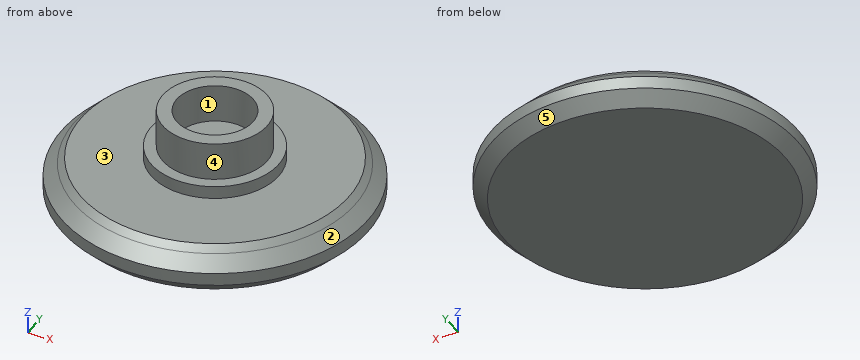
```python
from build123d import *

# Parameters (mm, degrees)
F0_R     = 12
F0_R_2   = 11
F0_R_3   = 5
F0_R_4   = 4.1
F0_R_5   = 3
F1_DEPTH = 2
F2_DEPTH = 3.5
F3_SIZE  = 0.99999
F4_DEPTH = 4.5
F5_DEPTH = 7.5
F6_SIZE  = 1
F7_SIZE  = 0.5


# Not quite as in the source:
# - a fillet or chamfer is up to 0.001 mm smaller than in the source, because OpenCascade refuses the exact size


with BuildPart() as f1:
    # F0 (on Top) → F1 (new body)
    with BuildSketch(Plane.XY):
        Circle(F0_R)
        Circle(F0_R_2, mode=Mode.SUBTRACT)
        Circle(F0_R_2)
        Circle(F0_R_3, mode=Mode.SUBTRACT)
        Circle(F0_R_3)
        Circle(F0_R_4, mode=Mode.SUBTRACT)
        Circle(F0_R_4)
        Circle(F0_R_5, mode=Mode.SUBTRACT)
        Circle(F0_R_5)
    extrude(amount=F1_DEPTH)

    # F0 (on Top) → F2 (join)
    with BuildSketch(Plane.XY):
        Circle(F0_R_2)
        Circle(F0_R_3, mode=Mode.SUBTRACT)
        Circle(F0_R_3)
        Circle(F0_R_4, mode=Mode.SUBTRACT)
        Circle(F0_R_4)
        Circle(F0_R_5, mode=Mode.SUBTRACT)
        Circle(F0_R_5)
    extrude(amount=F2_DEPTH)

    # F3 (size 1 in the source; OpenCascade refuses exactly that, so slightly less here)
    f3_edges = [f1.edges().sort_by_distance(p)[0] for p in [
        (-11, 0, 2),
    ]]
    chamfer(f3_edges, length=F3_SIZE)

    # F0 (on Top) → F4 (join)
    with BuildSketch(Plane.XY):
        Circle(F0_R_3)
        Circle(F0_R_4, mode=Mode.SUBTRACT)
        Circle(F0_R_4)
        Circle(F0_R_5, mode=Mode.SUBTRACT)
        Circle(F0_R_5)
    extrude(amount=F4_DEPTH)

    # F0 (on Top) → F5 (join)
    with BuildSketch(Plane.XY):
        Circle(F0_R_4)
        Circle(F0_R_5, mode=Mode.SUBTRACT)
    extrude(amount=F5_DEPTH)

    # F6
    f6_edges = [f1.edges().sort_by_distance(p)[0] for p in [
        (-12, 0, 0),
    ]]
    chamfer(f6_edges, length=F6_SIZE)

    # F7
    f7_edges = [f1.edges().sort_by_distance(p)[0] for p in [
        (-11, 0, 3.5),
    ]]
    chamfer(f7_edges, length=F7_SIZE)


solid = f1.part
```
Geometry: final body of the model. Coordinates: model frame, mm. Face numbers are marked on the shaded views. A direction names the side the tool comes from. Round coordinates to 2 decimals unless told otherwise and drop trailing zeros. Order: outer loops, then holes, each group sorted by start corner. A loop starts at its lowest first (then second) coordinate and runs counter-clockwise, first axis right, second up. Notation, with made-up numbers: (21, 56.25) - (70, 56.25) arc R30 cw to (70, 85.25) - close; hole circle Ø6 at (33, -37). An arc over 180 degrees is marked (long way). Use CSV: the item, a comma, the result in double quotes. Start each with the question number.
Q1. Access query for the marked faces 4 and 5. Directions: +Z, -Z, +X, -X, +Y, -Y. A direction counts if a zero-diameter tool reaches every point of the face in a straight line with its end or side. Return the directions, or none.
Q2. Material intervals for line 1 along X through (y, z) = (0, 6.4); line 2 along Z through (x, y) = (4.75, -4.5), sorted ascending. Write a range as from..to.
Q3. Section query D-D (z = 4). Return loops of the section in (x, y).
Q4. Mould query, pull axis Y, two halves, no side actions, for the marked faces 1, 2 and 3. Classes: +Y half, -Y half, draft (parallel to the pull), parting line (faces both ways), or undercut.
Q5. Section query B-B (z = 6.75). Return loops of the section in (x, y), and give its area (3 significant figures).
Q6. First-contact query: pin 1 (3.5 mm diameter, centred on x = 0, y = 0, fed in from +Z); pin 2 (2 mm diameter, centred on x = -7, y = 7, fed in from +Z); pin 3 (4 mm diameter, centred on x = -2.5, z = 2, fed in from +Y). Flat tips, straight axial feed; report the tip coordinate or a pass-through.
Result set:
1,face 4,"+Z"
1,face 5,"-Z"
2,line 1,"x = -4.1..-3, 3..4.1"
2,line 2,"z = 0..3.5"
3,outline,"circle Ø10 at (0, 0)"
4,face 1,"undercut"
4,face 2,"parting line"
4,face 3,"draft"
5,outline,"circle Ø8.2 at (0, 0); hole circle Ø6 at (0, 0)"
5,area,"24.5 mm2"
6,pin 1,"stops at z = 4.5"
6,pin 2,"stops at z = 3.5"
6,pin 3,"stops at y = 11.99"
